```python
from build123d import *

# Parameters (mm, degrees)
F1_DEPTH = 6
F2_R     = 1.05
F3_DEPTH = 1.5
F4_R     = 1.075
F5_DEPTH = 5
F6_R     = 0.5


with BuildPart() as f1:
    # F0 (on Front) → F1 (new body)
    with BuildSketch(Plane.XZ):
        Polygon((-2.85, -10), (2.85, -10), (2.85, 10), (1.00367, 10), (-2.85, 7), align=None)
    extrude(amount=F1_DEPTH)

    # F2 (on face) → F3 (cut)
    with BuildSketch(Plane(origin=(-2.85, 0, 0), x_dir=(0, -1, 0), z_dir=(-1, 0, 0))):
        with Locations((3, -4)):
            Circle(F2_R)
        with Locations((3, 3.25)):
            Circle(F2_R)
    extrude(amount=-F3_DEPTH, mode=Mode.SUBTRACT)

    # F4 (on face) → F5 (cut)
    with BuildSketch(Plane(origin=(0, 0, -10), x_dir=(1, 0, 0), z_dir=(0, 0, -1))):
        with Locations((-0.15, 3)):
            Circle(F4_R)
    extrude(amount=-F5_DEPTH, mode=Mode.SUBTRACT)

    # F6
    f6_edges = [f1.edges().sort_by_distance(p)[0] for p in [
        (2.85, -3, 10),
        (-2.85, -3, 7),
        (1.00367, -3, 10),
    ]]
    fillet(f6_edges, radius=F6_R)


solid = f1.part
```
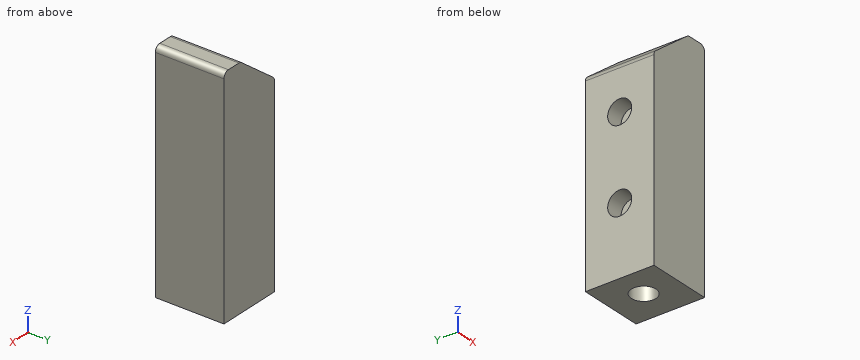
Geometry check sheet. Reference: the model listing, model coordinates, mm. Coordinates: 2 decimals unless noted, no trailing zeros. Order: outer loops, then holes, each group sorted by start corner. A loop starts at its lowest first (then second) coordinate and runs counter-clockwise, first axis right, second up.
Q1. Depth check by flat-ended pin: pin 1 Ø0.6 at (y, z) = (-3.5, -4.5) entering from -X. Enter the tip coordinate at first touch or a pass-through.
Reply:
pin 1: stops at x = -1.35
Q2. Sectioned sample at A-A on z = 3.25. Record the cut outline in (x, y).
Reply:
outline: (-2.85, -6) - (2.85, -6) - (2.85, 0) - (-2.85, 0) - (-2.85, -1.95) - (-1.35, -1.95) - (-1.35, -4.05) - (-2.85, -4.05) - close
Q3. Sectioned sample at B-B on x = -0.3. Record the cut outline in (y, z).
Reply:
outline: (-6, -10) - (-4.06, -10) - (-4.06, -5) - (-1.94, -5) - (-1.94, -10) - (0, -10) - (0, 8.99) - (-6, 8.99) - close
Q4. Sectioned sample at C-C on y = -3. Record the cut outline in (x, z) (3 decimals).
Reply:
outline: (-2.85, -10) - (-1.225, -10) - (-1.225, -5) - (0.925, -5) - (0.925, -10) - (2.85, -10) - (2.85, 9.5) arc R0.5 ccw to (2.35, 10) - (1.175, 10) arc R0.5 ccw to (0.868, 9.895) - (-2.657, 7.15) arc R0.5 ccw to (-2.85, 6.756) - (-2.85, 4.3) - (-1.35, 4.3) - (-1.35, 2.2) - (-2.85, 2.2) - (-2.85, -2.95) - (-1.35, -2.95) - (-1.35, -5.05) - (-2.85, -5.05) - close
Q5. Thickness scan on probe 1 along X at (y, z) = (-3, -7.7) (3 decimals); probe 2 along Y at (x, z) = (-0.15, -7.25) (3 decimals); probe 3 along Z at (x, y) = (-2.3, -3). Record the ranges inside material, lowest first.
Reply:
probe 1: x = -2.85 to -1.225, 0.925 to 2.85
probe 2: y = -6 to -4.075, -1.925 to 0
probe 3: z = -10 to -5.05, -2.95 to 2.2, 4.3 to 7.43
